from build123d import *

# Parameters (mm, degrees)
F1_DEPTH = 12.7
F2_R     = 3.175
F3_DEPTH = 110.6302371448
F5_R     = 7.9375
F5_R_2   = 3.175
F6_DEPTH = 104.2802371448


with BuildPart() as f1:
    # F0 (on Front) → F1 (new body, symmetric)
    with BuildSketch(Plane.XZ):
        Polygon((113.1007601121, 25.4), (5.3989366664, 25.4), (0, 0), (113.1007601121, 0), align=None)
    extrude(amount=F1_DEPTH, both=True)

    # F2 (on face) → F3 (cut, through all)
    with BuildSketch(Plane(origin=(0, 0, 0), x_dir=(0, -1, 0), z_dir=(-0.9781476007, 0, 0.2079116908))):
        with Locations((0, 12.9837255548)):
            Circle(F2_R)
    extrude(amount=-F3_DEPTH, mode=Mode.SUBTRACT)

    # F5 (on offset) → F6 (cut, through all)
    with BuildSketch(Plane(origin=(6.2112372647, 0, -1.3202392367), x_dir=(0, -1, 0), z_dir=(-0.9781476007, 0, 0.2079116908))):
        with Locations((0, 12.9837255548)):
            Circle(F5_R)
        with Locations((0, 12.9837255548)):
            Circle(F5_R_2, mode=Mode.SUBTRACT)
    extrude(amount=-F6_DEPTH, mode=Mode.SUBTRACT)


solid = f1.part
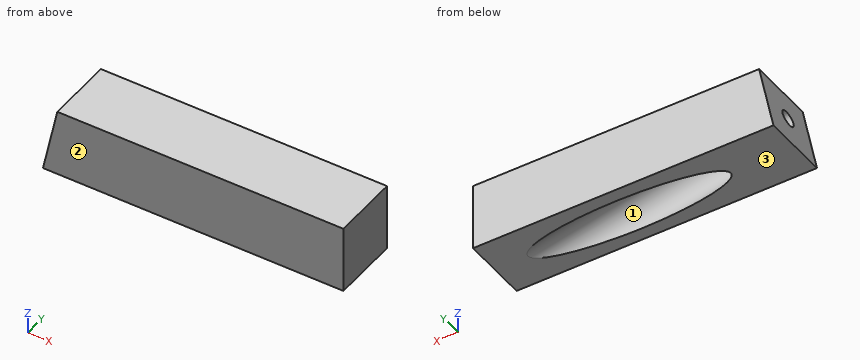
Geometry: final body of the model. Coordinates: model frame, mm. Face numbers are marked on the shaded views. Round coordinates to 2 decimals unless told otherwise and drop trailing zeros. Loops run counter-clockwise (first coordinate to the right, second up) from the corner with the lowest first, then second, coordinate; pieces in that order, holes last.
Q1. Section D-D on y = 9.25. Return loops of the section in (x, z).
Q2. Material intervals for L1, parallel to X at y = 8.25, z = 11.25; L2, parallel to Y at x = 60, z = 6; L3, parallel to Z at x = 96.5, y = -3.25, sorted ascending.
Q3. Section B-B on y = -6.25. Return loops of the section in (x, z).
Q4. Pull-direction query (Z, two-part tool) for the marked faces 1, 2 and 3; classes: released by +Z, released by -Z, zero draft, split by the parting line, or undercut.
Q5. Section C-C on z = 20.5. Return loops of the section in (x, y), plus the area to 3 significant figures.
Q6. Pin query (flat end, axial travel): P1, Ø8, axis at y = 4.5, z = 6.5, coming from the -X side; P2, Ø3, axis at y = 9.5, z = 17.5, coming from the -X side. Return the tip coordinate at first contact, or that it passes through.
Q7. Section A-A on y = -1.75. Return loops of the section in (x, z).
Evaluation:
1. outline: (0, 0) - (113.1, 0) - (113.1, 25.4) - (5.4, 25.4) - close
2. L1: x = 2.39 to 113.1
2. L2: y = -12.7 to -5.85, 5.85 to 12.7
2. L3: z = 0.17 to 25.4
3. outline: (0, 0) - (38.91, 0) - (7.89, 6.59) - (9.93, 16.17) - (85.98, 0) - (113.1, 0) - (113.1, 25.4) - (5.4, 25.4) - close
4. face 1: undercut
4. face 2: zero draft
4. face 3: released by -Z
5. outline: (4.36, -12.7) - (113.1, -12.7) - (113.1, 12.7) - (4.36, 12.7) - close
5. area: 2,760 mm2
6. P1: stops at x = 0.53
6. P2: stops at x = 3.4
7. outline: (0, 0) - (25.21, 0) - (7.3, 3.81) - (8.36, 8.79) - (2.15, 10.11) - close; (3.25, 15.29) - (9.46, 13.97) - (10.52, 18.95) - (99.69, 0) - (113.1, 0) - (113.1, 25.4) - (5.4, 25.4) - close
